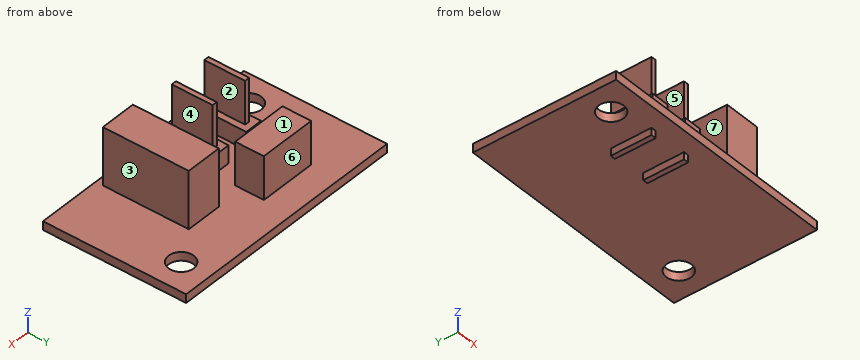
from build123d import *

# Parameters (mm, degrees)
SKETCH1_W           = 34
SKETCH1_H           = 20
BOSS_EXTRUDE1_DEPTH = 0.6
SKETCH2_W           = 2.5
SKETCH2_H           = 7.5
BOSS_EXTRUDE2_DEPTH = 2.5
SKETCH3_W           = 0.7
SKETCH3_H           = 5.7
BOSS_EXTRUDE3_DEPTH = 6
SKETCH4_W           = 0.7
SKETCH4_H           = 5.7
BOSS_EXTRUDE4_DEPTH = 1
SKETCH6_W           = 5.08
SKETCH6_H           = 12
BOSS_EXTRUDE5_DEPTH = 8
SKETCH7_W           = 8
SKETCH7_H           = 4
BOSS_EXTRUDE6_DEPTH = 6
SKETCH8_R           = 1.75
CUT_EXTRUDE1_DEPTH  = 22.476731595


with BuildPart() as part:
    # Sketch1 → Boss-Extrude1 (new, symmetric)
    with BuildSketch(Plane.XY):
        Rectangle(SKETCH1_W, SKETCH1_H)
    extrude(amount=BOSS_EXTRUDE1_DEPTH, both=True)

    # Sketch2 → Boss-Extrude2 (add)
    with BuildSketch(Plane.XY.offset(0.6)):
        with Locations((-7.75, -4.75)):
            Rectangle(SKETCH2_W, SKETCH2_H)
        with Locations((-2.25, -4.75)):
            Rectangle(SKETCH2_W, SKETCH2_H)
    extrude(amount=BOSS_EXTRUDE2_DEPTH)

    # Sketch3 → Boss-Extrude3 (add)
    with BuildSketch(Plane.XY.offset(3.1)):
        with Locations((-7.75, -4.75)):
            Rectangle(SKETCH3_W, SKETCH3_H)
        with Locations((-2.25, -4.75)):
            Rectangle(SKETCH3_W, SKETCH3_H)
    extrude(amount=BOSS_EXTRUDE3_DEPTH)

    # Sketch4 → Boss-Extrude4 (add)
    with BuildSketch(Plane(origin=(0, 0, -0.6), x_dir=(-1, 0, 0), z_dir=(0, 0, -1))):
        with Locations((7.75, -4.75)):
            Rectangle(SKETCH4_W, SKETCH4_H)
        with Locations((2.25, -4.75)):
            Rectangle(SKETCH4_W, SKETCH4_H)
    extrude(amount=BOSS_EXTRUDE4_DEPTH)

    # Sketch6 → Boss-Extrude5 (add)
    with BuildSketch(Plane.XY.offset(0.6)):
        with Locations((5.54, -3)):
            Rectangle(SKETCH6_W, SKETCH6_H)
    extrude(amount=BOSS_EXTRUDE5_DEPTH)

    # Sketch7 → Boss-Extrude6 (add)
    with BuildSketch(Plane.XY.offset(0.6)):
        with Locations((-5, 4)):
            Rectangle(SKETCH7_W, SKETCH7_H)
    extrude(amount=BOSS_EXTRUDE6_DEPTH)

    # Sketch8 → Cut-Extrude1 (cut, through all)
    with BuildSketch(Plane.XY.offset(0.6)):
        with Locations((-13, -6)):
            Circle(SKETCH8_R)
        with Locations((13, 6)):
            Circle(SKETCH8_R)
    extrude(amount=-CUT_EXTRUDE1_DEPTH, mode=Mode.SUBTRACT)


solid = part.part
Could you check a few things on this model? Use its own coordinates, in mm. Face numbers are marked on the shaded views. A direction names the side the tool comes from. Give positions to 0.01 mm unless a question says otherwise; leave off trailing zeros. Order: outer loops, then holes, each group sorted by start corner. A loop starts at its lowest first (then second) coordinate and runs counter-clockwise, first axis right, second up. Notation, with made-up numbers: (19, 76) -> (63, 76) arc R11 ccw to (63, 85) -> close; hole circle Ø6 at (53.5, -18.75). An arc over 180 degrees is marked (long way). Answer in a Markdown table with one row per item. Add a question column.
Item 1: Please list where these lines run through material, in increasing order: probe 1 along X at (y, z) = (-6.5, 6.5); probe 2 along X at (y, z) = (-7.5, 2); probe 3 along Y at (x, z) = (-13, 0).
Item 2: Imagine slicing it at C-C (z = 2.5). List the corners of the cut face in (x, y) for me.
Item 3: Imagine slicing it at A-A (z = 7). List the corners of the cut face in (x, y) for me, and give its area (3 significant figures).
Item 4: I'm going to push flat-ended pins straight in: P1, Ø1.5, axis at x = 3, z = 5.5, coming from the -Y side; P2, Ø1.2, axis at y = -3.5, z = 2, coming from the +X side; P3, Ø5, axis at x = -7, z = 5, coming from the -Y side; P4, Ø3, axis at x = -13, y = -6, coming from the -Z side. Where does each tip first touch, or does it pass through?
Item 5: We'd pull the mould along X, two halves only. Please class the marked faces 1, 2, 3 and 4: pulls with the +X half, pulls with the -X half, needs draft (parallel to the pull), parting line crosses it, or undercut.
Item 6: For the marked faces 5, 6 and 7, which set-ups out of +Z, -Z, +X, -X, +Y, -Y let a thin tool reach every point of the face, with its end or its side?
Item 7: Imagine slicing it at B-B (x = 13). List the corners of the cut face in (y, z) for me.
Item 8: Imagine slicing it at D-D (y = 1). List the corners of the cut face in (x, z) for me.
Result:
| question | item | result |
|---|---|---|
| 1 | probe 1 | -8.1 to -7.4, -2.6 to -1.9, 3 to 8.08 |
| 1 | probe 2 | -9 to -6.5, -3.5 to -1, 3 to 8.08 |
| 1 | probe 3 | -10 to -7.75, -4.25 to 10 |
| 2 | outline | (-9, -8.5) -> (-6.5, -8.5) -> (-6.5, -1) -> (-9, -1) -> close; (-9, 2) -> (-1, 2) -> (-1, 6) -> (-9, 6) -> close; (-3.5, -8.5) -> (-1, -8.5) -> (-1, -1) -> (-3.5, -1) -> close; (3, -9) -> (8.08, -9) -> (8.08, 3) -> (3, 3) -> close |
| 3 | outline | (-8.1, -7.6) -> (-7.4, -7.6) -> (-7.4, -1.9) -> (-8.1, -1.9) -> close; (-2.6, -7.6) -> (-1.9, -7.6) -> (-1.9, -1.9) -> (-2.6, -1.9) -> close; (3, -9) -> (8.08, -9) -> (8.08, 3) -> (3, 3) -> close |
| 3 | area | 68.9 mm2 |
| 4 | P1 | y = -9 |
| 4 | P2 | x = 8.08 |
| 4 | P3 | y = -8.5 |
| 4 | P4 | through |
| 5 | face 1 | needs draft |
| 5 | face 2 | undercut |
| 5 | face 3 | pulls with the +X half |
| 5 | face 4 | undercut |
| 6 | face 5 | +Z, -Y |
| 6 | face 6 | +Z, +X, -X, +Y |
| 6 | face 7 | +Z, +Y, -Y |
| 7 | outline | (-10, -0.6) -> (4.25, -0.6) -> (4.25, 0.6) -> (-10, 0.6) -> close; (7.75, -0.6) -> (10, -0.6) -> (10, 0.6) -> (7.75, 0.6) -> close |
| 8 | outline | (-17, -0.6) -> (17, -0.6) -> (17, 0.6) -> (8.08, 0.6) -> (8.08, 8.6) -> (3, 8.6) -> (3, 0.6) -> (-17, 0.6) -> close |
